from build123d import *

# Parameters (mm, degrees)
F0_W     = 210
F0_H     = 15
F1_DEPTH = 10
F3_DEPTH = 10


with BuildPart() as f1:
    # F0 (on Top) → F1 (new body)
    with BuildSketch(Plane.XY):
        Rectangle(F0_W, F0_H)
    extrude(amount=F1_DEPTH)

    # F2 (on face) → F3 (cut)
    with BuildSketch(Plane.XZ.offset(7.5)):
        with BuildLine():
            ThreePointArc((68, 5), (70, 3), (72, 5))
            Line((72, 5), (68, 5))
        make_face()
        with BuildLine():
            Line((68, 5), (72, 5))
            ThreePointArc((72, 5), (70, 7), (68, 5))
        make_face()
        with BuildLine():
            ThreePointArc((-72, 5), (-70, 3), (-68, 5))
            Line((-68, 5), (-72, 5))
        make_face()
        with BuildLine():
            Line((-72, 5), (-68, 5))
            ThreePointArc((-68, 5), (-70, 7), (-72, 5))
        make_face()
        with BuildLine():
            ThreePointArc((-42, 5), (-40, 3), (-38, 5))
            Line((-38, 5), (-42, 5))
        make_face()
        with BuildLine():
            Line((-42, 5), (-38, 5))
            ThreePointArc((-38, 5), (-40, 7), (-42, 5))
        make_face()
        with BuildLine():
            ThreePointArc((38, 5), (40, 3), (42, 5))
            Line((42, 5), (38, 5))
        make_face()
        with BuildLine():
            Line((38, 5), (42, 5))
            ThreePointArc((42, 5), (40, 7), (38, 5))
        make_face()
    extrude(amount=-F3_DEPTH, mode=Mode.SUBTRACT)


solid = f1.part
Read the model definition and answer for the solid it produces. Units are mm, in the model's axes. A direction names the side the tool comes from. Coordinates: 2 decimals unless noted, no trailing zeros. Loops run counter-clockwise (first coordinate to the right, second up) from the corner with the lowest first, then second, coordinate; pieces in that order, holes last. Notation, with made-up numbers: (10.5, -30.75) -> (37.5, -30.75) arc R22 ccw to (37.5, 4.25) -> close; hole circle Ø7 at (-35.75, 17). An arc over 180 degrees is marked (long way). Write item = value, one per line. Start each with the question number.
1) The part is cut by section B-B, the plane z = 5. Determine the outline of the cut face in (x, y), plus the area to 3 significant figures.
2) The part is cut by section C-C, the plane x = 40. Determine the outline of the cut face in (y, z).
3) Find the intervals of material crossed by L1, parallel to Z at x = -70, y = -4; L2, parallel to X at y = -5.25, z = 3.5; L3, parallel to X at y = 1.5, z = 6, in increasing order. Write a range as from..to.
4) The mould has two halves that part along Z. Classify faces 3 (the face through (70, 2.5, 5)), 4 (the face through (-1, -7.5, 5)), 5 (the face through (-1, 0, 0)), 6 (the face through (-1, 0, 10)): pulls with the +Z half, pulls with the -Z half, needs draft (parallel to the pull), parting line crosses it, or undercut.
5) Given P1, Ø1.2, axis at x = -69, z = 4.5, coming from the -Y side; P2, Ø3, axis at x = 39, z = 5.5, coming from the -Y side, each flat-ended and moving along its own axis, determine where each tip first touches the part or whether it passes through.
6) For faces 1 (the face through (-68.092, -2.57, 5.601)), 2 (the face through (105, 0, 5)), determine the directions among +Z, -Z, +X, -X, +Y, -Y from which every point of the face is accessible in a straight line to the end or side of a thin tool.
7) The part is cut by section A-A, the plane y = -4. Determine the outline of the cut face in (x, z).
Result:
q1.outline = (-105, -7.5) -> (-72, -7.5) -> (-72, 2.5) -> (-68, 2.5) -> (-68, -7.5) -> (-42, -7.5) -> (-42, 2.5) -> (-38, 2.5) -> (-38, -7.5) -> (38, -7.5) -> (38, 2.5) -> (42, 2.5) -> (42, -7.5) -> (68, -7.5) -> (68, 2.5) -> (72, 2.5) -> (72, -7.5) -> (105, -7.5) -> (105, 7.5) -> (-105, 7.5) -> close
q1.area = 2,990 mm²
q2.outline = (-7.5, 0) -> (7.5, 0) -> (7.5, 10) -> (-7.5, 10) -> (-7.5, 7) -> (2.5, 7) -> (2.5, 3) -> (-7.5, 3) -> close
q3.L1 = 0..3, 7..10
q3.L2 = -105..-71.32, -68.68..-41.32, -38.68..38.68, 41.32..68.68, 71.32..105
q3.L3 = -105..-71.73, -68.27..-41.73, -38.27..38.27, 41.73..68.27, 71.73..105
q4.face_3 = undercut
q4.face_4 = needs draft
q4.face_5 = pulls with the -Z half
q4.face_6 = pulls with the +Z half
q5.P1 = 2.5
q5.P2 = -7.5
q6.face_1 = -Y
q6.face_2 = +Z, -Z, +X, +Y, -Y
q7.outline = (-105, 0) -> (105, 0) -> (105, 10) -> (-105, 10) -> close; hole circle Ø4 at (-70, 5); hole circle Ø4 at (-40, 5); hole circle Ø4 at (40, 5); hole circle Ø4 at (70, 5)
